```python
from build123d import *

# Parameters (mm, degrees)
SKETCH1_W           = 50.8
SKETCH1_H           = 25.4
SKETCH1_W_2         = 47.625
SKETCH1_H_2         = 22.225
BOSS_EXTRUDE1_DEPTH = 457.2
SKETCH2_R           = 12.7
CUT_EXTRUDE1_DEPTH  = 25.4
SKETCH4_R           = 12.7
CUT_EXTRUDE2_DEPTH  = 25.4
SKETCH5_R           = 12.7
CUT_EXTRUDE5_DEPTH  = 25.4


with BuildPart() as part:
    # Sketch1 → Boss-Extrude1 (new body)
    with BuildSketch(Plane.XY):
        with Locations((25.4, 12.7)):
            Rectangle(SKETCH1_W, SKETCH1_H)
        with Locations((25.4, 12.7)):
            Rectangle(SKETCH1_W_2, SKETCH1_H_2, mode=Mode.SUBTRACT)
    extrude(amount=BOSS_EXTRUDE1_DEPTH)

    # Sketch2 → Cut-Extrude1 (cut)
    with BuildSketch(Plane(origin=(0, 25.4, 0), x_dir=(1, 0, 0), z_dir=(0, 1, 0))):
        with Locations(Location((25.4, -381, 0), (0, 0, 270))):
            Circle(SKETCH2_R)
    extrude(amount=-CUT_EXTRUDE1_DEPTH, mode=Mode.SUBTRACT)

    # Sketch4 → Cut-Extrude2 (cut)
    with BuildSketch(Plane(origin=(0, 25.4, 0), x_dir=(1, 0, 0), z_dir=(0, 1, 0))):
        with Locations(Location((25.4, -76.2, 0), (0, 0, 270))):
            Circle(SKETCH4_R)
    extrude(amount=-CUT_EXTRUDE2_DEPTH, mode=Mode.SUBTRACT)

    # Sketch5 → Cut-Extrude5 (cut)
    with BuildSketch(Plane(origin=(0, 25.4, 0), x_dir=(1, 0, 0), z_dir=(0, 1, 0))):
        with Locations(Location((31.75, -228.6, 0), (0, 0, 270))):
            Circle(SKETCH5_R)
    extrude(amount=-CUT_EXTRUDE5_DEPTH, mode=Mode.SUBTRACT)


solid = part.part
```
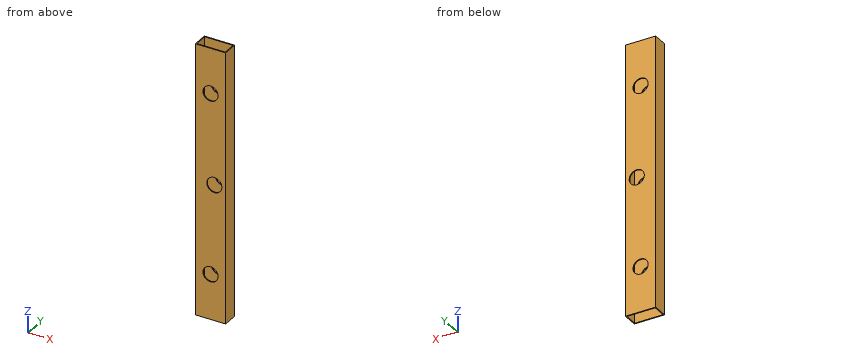
The listing builds one solid part. Answer for the finished solid, in the listing's coordinates (mm). Give positions to 0.01 mm unless a question says otherwise; leave off trailing zeros. Loops run counter-clockwise (first coordinate to the right, second up) from the corner with the lowest first, then second, coordinate; pieces in that order, holes last. Notation, with made-up numbers: (19.5, 33) - (40.5, 33) arc R20 cw to (40.5, 64) - close; hole circle Ø2 at (39.25, 7.5). An arc over 180 degrees is marked (long way). Return JSON: item names as keys, results as strings. Group by question number.
1. Find section B-B (y = 12). Write down the section's boundary in (x, z), then the cut area to 3 significant figures.
2. Find section C-C (x = 25.4). State how many separate pieces and enclosed holes the cut face has, then the cut area to 3 significant figures.
3. Straight lines are drawn through the part: line 1 (X direction, y = 23.5, z = 315); line 2 (Y direction, x = 45.5, z = 190.5); line 3 (X direction, y = 1.1, z = 76.2). For each, find the intervals that lie inside material, in ascending order. Write a range as [from, to].
4. Find section A-A (z = 340). Write down the section's boundary in (x, y).
Verdict:
{
 "1": {"outline": "(0, 0) - (1.59, 0) - (1.59, 457.2) - (0, 457.2) - close; (49.21, 0) - (50.8, 0) - (50.8, 457.2) - (49.21, 457.2) - close", "area": "1,450 mm^2"},
 "2": {"separate pieces": "8", "enclosed holes": "0", "area": "1,220 mm^2"},
 "3": {"line 1": "x = [0, 1.59], [49.21, 50.8]", "line 2": "y = [0, 1.59], [23.81, 25.4]", "line 3": "x = [0, 12.7], [38.1, 50.8]"},
 "4": {"outline": "(0, 0) - (50.8, 0) - (50.8, 25.4) - (0, 25.4) - close; hole (1.59, 1.59) - (49.21, 1.59) - (49.21, 23.81) - (1.59, 23.81) - close"}
}
